Can you work these out from the drawing? Everything is in mm from the part's minimum corner. A direction names the side the tool comes from. Coordinates: 2 decimals unless noted, no trailing zeros. Write each loop counter-clockwise with the first axis right and the second up, starting at its lowest first coordinate (ties: lowest second). Pieces come first, ordered by that corner, then holes. Notation, with made-up numbers: M -33.75,80 L 7.25,80 A27 cw 7.25,117 Z; hole C -28,-3 d2. An arc over 180 degrees is marked long. Answer as a JSON object with one key per item and string values. Group by question number.
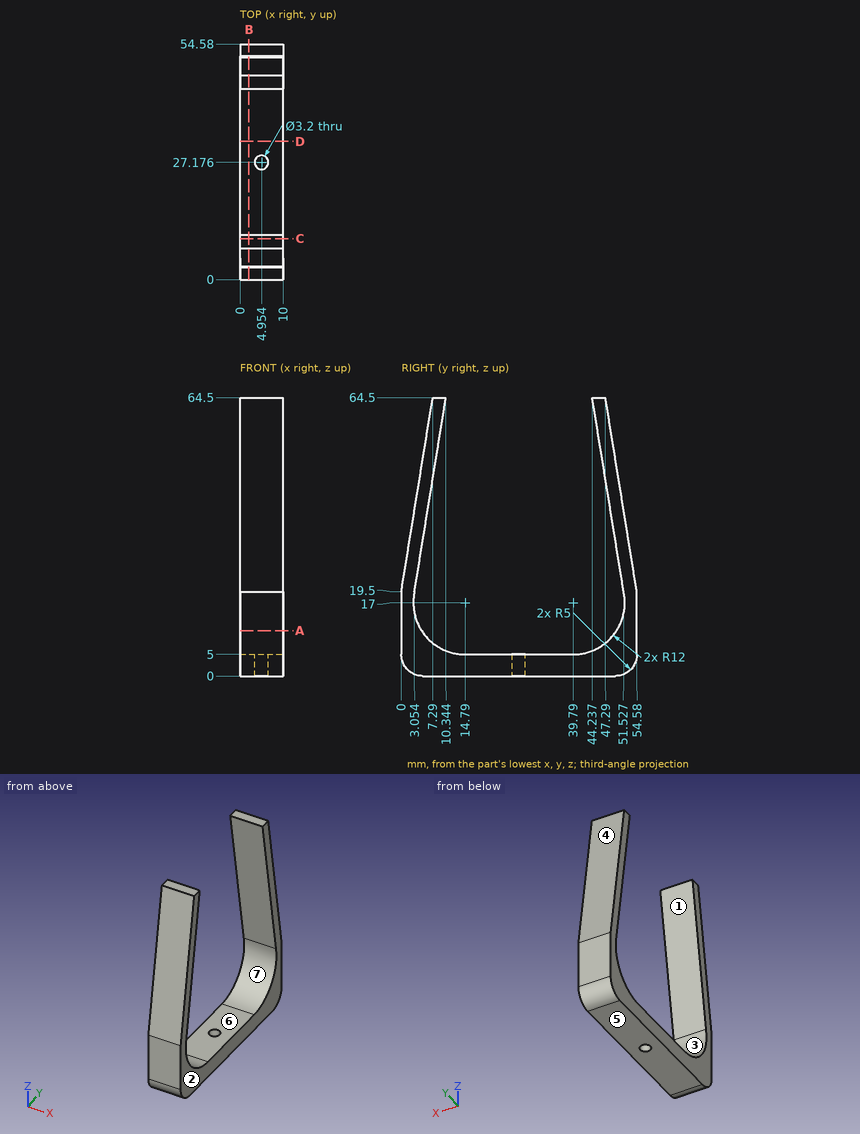
Q1. We'd pull the mould along Y, two halves only. Please class the marked faces 1, 2, 3 and 4: pulls with the +Y half, pulls with the -Y half, needs draft (parallel to the pull), parting line crosses it, or undercut.
Q2. If we section it at A-A on z = 10.5: List the corners of the cut face in (x, y) for me.
Q3. Will this pin go through, and if not, where does the flat tip stop? pin 1 (1.5 mm diameter, centred on x = 2, z = 51.5, fed in from +Y).
Q4. If we section it at B-B on x = 2: List the corners of the cut face in (y, z) for me.
Q5. If we section it at D-D on y = 32: List the corners of the cut face in (x, z) for me.
Q6. Please list where these lines run through material, in increasing order: L1, parallel to Y at x = 7.75, z = 17; L2, parallel to Y at x = 6.25, z = 22 (1 decimal); L3, parallel to Z at x = 8, y = 29.
Q7. On a 3-axis mill with a long thin cutter (end or side, diameter ignored), from which of +Z, -Z, +X, -X, +Y, -Y can I reach the whole of each face in a straight line? I mean the marked faces 5, 6 and 7. Say none if no direction works.
Q8. If we section it at C-C on y = 9.5: List the corners of the cut face in (x, z) for me, and give its area (3 significant figures).
Reply:
{
 "1": {"face 1": "undercut", "face 2": "needs draft", "face 3": "undercut", "face 4": "pulls with the +Y half"},
 "2": {"outline": "M 0,0 L 10,0 L 10,4.7 L 0,4.7 Z; M 0,49.88 L 10,49.88 L 10,54.58 L 0,54.58 Z"},
 "3": {"pin 1": "y = 49.52"},
 "4": {"outline": "M 0,5 A5 ccw 5,0 L 49.58,0 A5 ccw 54.58,5 L 54.58,19.5 L 47.29,64.5 L 44.24,64.5 L 51.53,19.5 A12 cw 39.79,5 L 14.79,5 A12 cw 3.05,19.5 L 10.34,64.5 L 7.29,64.5 L 0,19.5 Z"},
 "5": {"outline": "M 0,0 L 10,0 L 10,5 L 0,5 Z"},
 "6": {"L1": "0 to 2.79, 51.79 to 54.58", "L2": "0.4 to 3.5, 51.1 to 54.2", "L3": "0 to 5"},
 "7": {"face 5": "-Z, +X, -X, +Y, -Y", "face 6": "+Z, +X, -X", "face 7": "+X, -X"},
 "8": {"outline": "M 0,0 L 10,0 L 10,6.23 L 0,6.23 Z; M 0,59.29 L 10,59.29 L 10,64.5 L 0,64.5 Z", "area": "114 mm^2"}
}
